from build123d import *

# Parameters (mm, degrees)
SKETCH1_R                = 3.2
EXTRUDE1_DEPTH           = 3
SKETCH2_W                = 15
SKETCH2_H                = 15
SKETCH2_R                = 2.65
EXTRUDE2_DEPTH           = 1.6
SKETCH3_W                = 0.6
SKETCH3_H                = 0.6
EXTRUDE3_DEPTH           = 6
SKETCH4_R                = 0.625
EXTRUDE4_DEPTH           = 1.25
EXTRUDE4_DRAFT           = 5
EXTRUDE4_PROFILE_2_DEPTH = 1.25
EXTRUDE4_PROFILE_2_DRAFT = 5
EXTRUDE4_PROFILE_3_DEPTH = 1.25
EXTRUDE4_PROFILE_3_DRAFT = 5
EXTRUDE4_PROFILE_4_DEPTH = 1.25
EXTRUDE4_PROFILE_4_DRAFT = 5
CUT_EXTRUDE1_DEPTH       = 0.2


with BuildPart() as part:
    # Sketch1 → Extrude1 (new body)
    with BuildSketch(Plane.XY):
        with BuildLine():
            Line((-5.1, 7.6), (5.1, 7.6))
            ThreePointArc((5.1, 7.6), (5.832233047, 5.832233047), (7.6, 5.1))
            Line((7.6, 5.1), (7.6, -5.1))
            ThreePointArc((7.6, -5.1), (5.832233047, -5.832233047), (5.1, -7.6))
            Line((5.1, -7.6), (-5.1, -7.6))
            ThreePointArc((-5.1, -7.6), (-5.832233047, -5.832233047), (-7.6, -5.1))
            Line((-7.6, -5.1), (-7.6, 5.1))
            ThreePointArc((-7.6, 5.1), (-5.832233047, 5.832233047), (-5.1, 7.6))
        make_face()
        Circle(SKETCH1_R, mode=Mode.SUBTRACT)
    extrude(amount=EXTRUDE1_DEPTH)

    # Sketch2 → Extrude2 (add)
    with BuildSketch(Plane.XY.offset(3)):
        Rectangle(SKETCH2_W, SKETCH2_H)
        Circle(SKETCH2_R, mode=Mode.SUBTRACT)
    extrude(amount=EXTRUDE2_DEPTH)

    # Sketch3 → Extrude3 (add)
    with BuildSketch(Plane.XY.offset(4.6)):
        with Locations((-6.26, 6.26)):
            Rectangle(SKETCH3_W, SKETCH3_H)
        with Locations((6.26, 6.26)):
            Rectangle(SKETCH3_W, SKETCH3_H)
        with Locations((-6.26, -6.26)):
            Rectangle(SKETCH3_W, SKETCH3_H)
    extrude(amount=EXTRUDE3_DEPTH)


with BuildPart() as extrude4_tool:
    # Sketch4 → Extrude4 (with draft: the straight prism first)
    with BuildSketch(Plane.XY.offset(4.6)):
        with Locations((-4.2, -6.5)):
            Circle(SKETCH4_R)
    extrude(amount=EXTRUDE4_DEPTH)
    # Extrude4: the draft: its side faces are tilted about the plane it starts from
    extrude4_sides = [extrude4_tool.faces().sort_by_distance(p)[0] for p in [
        (-4.825, -6.5, 5.225),
    ]]
    draft(extrude4_sides, Plane.XY.offset(4.6), EXTRUDE4_DRAFT)


with BuildPart() as part_1:
    add(part.part)

    # Extrude4: add extrude4_tool
    add(extrude4_tool.part)


with BuildPart() as extrude4_profile_2_tool:
    # Sketch4 → Extrude4 profile 2 (with draft: the straight prism first)
    with BuildSketch(Plane.XY.offset(4.6)):
        with Locations((4.2, -6.5)):
            Circle(SKETCH4_R)
    extrude(amount=EXTRUDE4_PROFILE_2_DEPTH)
    # Extrude4 profile 2: the draft: its side faces are tilted about the plane it starts from
    extrude4_profile_2_sides = [extrude4_profile_2_tool.faces().sort_by_distance(p)[0] for p in [
        (3.575, -6.5, 5.225),
    ]]
    draft(extrude4_profile_2_sides, Plane.XY.offset(4.6), EXTRUDE4_PROFILE_2_DRAFT)


with BuildPart() as part_2:
    add(part_1.part)

    # Extrude4 profile 2: add extrude4_profile_2_tool
    add(extrude4_profile_2_tool.part)


with BuildPart() as extrude4_profile_3_tool:
    # Sketch4 → Extrude4 profile 3 (with draft: the straight prism first)
    with BuildSketch(Plane.XY.offset(4.6)):
        with Locations((-6.5, 4.2)):
            Circle(SKETCH4_R)
    extrude(amount=EXTRUDE4_PROFILE_3_DEPTH)
    # Extrude4 profile 3: the draft: its side faces are tilted about the plane it starts from
    extrude4_profile_3_sides = [extrude4_profile_3_tool.faces().sort_by_distance(p)[0] for p in [
        (-7.125, 4.2, 5.225),
    ]]
    draft(extrude4_profile_3_sides, Plane.XY.offset(4.6), EXTRUDE4_PROFILE_3_DRAFT)


with BuildPart() as part_3:
    add(part_2.part)

    # Extrude4 profile 3: add extrude4_profile_3_tool
    add(extrude4_profile_3_tool.part)


with BuildPart() as extrude4_profile_4_tool:
    # Sketch4 → Extrude4 profile 4 (with draft: the straight prism first)
    with BuildSketch(Plane.XY.offset(4.6)):
        with Locations((6.5, 4.2)):
            Circle(SKETCH4_R)
    extrude(amount=EXTRUDE4_PROFILE_4_DEPTH)
    # Extrude4 profile 4: the draft: its side faces are tilted about the plane it starts from
    extrude4_profile_4_sides = [extrude4_profile_4_tool.faces().sort_by_distance(p)[0] for p in [
        (5.875, 4.2, 5.225),
    ]]
    draft(extrude4_profile_4_sides, Plane.XY.offset(4.6), EXTRUDE4_PROFILE_4_DRAFT)


with BuildPart() as part_4:
    add(part_3.part)

    # Extrude4 profile 4: add extrude4_profile_4_tool
    add(extrude4_profile_4_tool.part)

    # Sketch5 → Cut-Extrude1 (cut)
    with BuildSketch(Plane(origin=(0, 0, 0), x_dir=(-1, 0, 0), z_dir=(0, 0, -1))):
        Polygon((-1.6, 7.6), (1.6, 7.6), (1.6, 7.1), (0.6, 7.1), (0, 6.5), (-0.6, 7.1), (-1.6, 7.1), align=None)
    extrude(amount=-CUT_EXTRUDE1_DEPTH, mode=Mode.SUBTRACT)


solid = part_4.part
Could you check a few things on this model? Use its own coordinates, in mm. A direction names the side the tool comes from. Give positions to 0.01 mm unless a question says otherwise; leave off trailing zeros. Write each loop counter-clockwise with the first axis right and the second up, starting at its lowest first coordinate (ties: lowest second). Pieces come first, ordered by that corner, then holes. Notation, with made-up numbers: (48, 67) - (62, 67) arc R36 cw to (62, 104) - close; hole circle Ø5 at (21, 19). An arc over 180 degrees is marked (long way). Use CSV: the item, a comma, the result in double quotes. Start each with the question number.
Item 1: For faces 4 (the face through (-5.852, 5.813, 1.479)), 5 (the face through (-5.813, -5.852, 1.479)), 6 (the face through (0, -7.5, 4)), 7 (the face through (0, 7, 0.2)), 8 (the face through (7, -7, 3)), which set-ups out of +Z, -Z, +X, -X, +Y, -Y let a thin tool reach every point of the face, with its end or its side?
Item 2: If I drill on line 1 along Y through (x, z) = (0, 1.5); line 2 along X through (y, z) = (6, 3.25); line 3 along Z through (x, y) = (-2.75, -0.25), over which ranges is the centre line in solid material (lowest first)?
Item 3: I'm going to push flat-ended pins straight in: pin 1 (0.5 mm diameter, centred on y = -6.5, z = 6, fed in from +X); pin 2 (0.7 mm diameter, centred on x = -6.5, z = 7.5, fed in from +Y); pin 3 (0.8 mm diameter, centred on y = -1, z = 4, fed in from +X); pin 4 (7 mm diameter, centred on x = -0.5, y = 1.5, fed in from -Z). Where does each tip first touch, or does it pass through?
Item 4: I want a section at D-D, the plane z = 5.25. Please give me the cut outline in (x, y), then the cut area to 3 significant figures.
Item 5: I want a section at A-A, the plane z = 9. Please give me the cut outline in (x, y).
Item 6: I want a section at C-C, the plane y = -1.25. Please give me the cut outline in (x, z), then the cut area to 3 significant figures.
Item 7: I want a section at B-B, the plane x = -0.25. Please give me the cut outline in (y, z).
Item 8: If we mould it in two halves opening along Y, with no side actions, what happens to faces 1 (the face through (-5.955, 4.372, 5.216)), 2 (the face through (4.126, -5.934, 5.216)), 3 (the face through (7.5, 0, 4))? For each: pulls with the +Y half, pulls with the -Y half, needs draft (parallel to the pull), parting line crosses it, or undercut.
Findings:
1,face 4,"-Z, -X, +Y"
1,face 5,"-Z, -X, -Y"
1,face 6,"+Z, +X, -X, -Y"
1,face 7,"-Z, +Y"
1,face 8,"-Z, +X, -Y"
2,line 1,"y = -7.6 to -3.2, 3.2 to 7.6"
2,line 2,"x = -7.5 to 7.5"
2,line 3,"z = 3 to 4.6"
3,pin 1,"stops at x = 4.72"
3,pin 2,"stops at y = 6.56"
3,pin 3,"stops at x = 7.5"
3,pin 4,"stops at z = 0"
4,outline,"circle Ø1.14 at (-6.5, 4.2); (-6.56, -6.56) - (-5.96, -6.56) - (-5.96, -5.96) - (-6.56, -5.96) - close; (-6.56, 5.96) - (-5.96, 5.96) - (-5.96, 6.56) - (-6.56, 6.56) - close; circle Ø1.14 at (-4.2, -6.5); circle Ø1.14 at (4.2, -6.5); circle Ø1.14 at (6.5, 4.2); (5.96, 5.96) - (6.56, 5.96) - (6.56, 6.56) - (5.96, 6.56) - close"
4,area,"5.14 mm2"
5,outline,"(-6.56, -6.56) - (-5.96, -6.56) - (-5.96, -5.96) - (-6.56, -5.96) - close; (-6.56, 5.96) - (-5.96, 5.96) - (-5.96, 6.56) - (-6.56, 6.56) - close; (5.96, 5.96) - (6.56, 5.96) - (6.56, 6.56) - (5.96, 6.56) - close"
6,outline,"(-7.6, 0) - (-2.95, 0) - (-2.95, 3) - (-2.34, 3) - (-2.34, 4.6) - (-7.5, 4.6) - (-7.5, 3) - (-7.6, 3) - close; (2.34, 3) - (2.95, 3) - (2.95, 0) - (7.6, 0) - (7.6, 3) - (7.5, 3) - (7.5, 4.6) - (2.34, 4.6) - close"
6,area,"44.4 mm2"
7,outline,"(-7.6, 0) - (-3.19, 0) - (-3.19, 3) - (-2.64, 3) - (-2.64, 4.6) - (-7.5, 4.6) - (-7.5, 3) - (-7.6, 3) - close; (2.64, 3) - (3.19, 3) - (3.19, 0) - (6.75, 0) - (6.75, 0.2) - (7.6, 0.2) - (7.6, 3) - (7.5, 3) - (7.5, 4.6) - (2.64, 4.6) - close"
8,face 1,"undercut"
8,face 2,"parting line crosses it"
8,face 3,"needs draft"
